Geometry: final body of the model. Coordinates: model frame, mm. A direction names the side the tool comes from. Round coordinates to 2 decimals unless told otherwise and drop trailing zeros. Write each loop counter-clockwise with the first axis right and the second up, starting at its lowest first coordinate (ties: lowest second). Pieces come first, ordered by that corner, then holes. Notation, with made-up numbers: M -5.5,8.25 L 19.5,8.25 A28 cw 19.5,32.25 Z; hole C -36.75,69 d9. An arc over 180 degrees is marked long. Answer as CSV lines item,"result". Start each with the question number.
Q1. Section query B-B on x = 9.75. Output: boundary loops of the cut face in (y, z), and give its area (3 significant figures).
Q2. First-contact query: pin 1 (1.6 mm diameter, centred on x = 5.5, y = 1.5, fed in from +Z); pin 2 (5 mm diameter, centred on x = 6.5, z = 3, fed in from +Y); pin 3 (6 mm diameter, centred on x = 6.5, z = 7.5, fed in from +Y); pin 4 (1.6 mm diameter, centred on y = 0.5, z = 6, fed in from +X). Flat tips, straight axial feed; report the tip coordinate or a pass-through.
Q3. Section query C-C on z = 12.5. Output: boundary loops of the cut face in (x, y).
Q4. Mould query, pull axis X, two halves, no side actions, for faces 1 (the flat face through (0, 0, 7)), 2 (the cylindrical face through (5.66, 0.89, 5.61)), 3 (the flat face through (7, 1.8, 7)). Classes: pulls with the +X half, pulls with the -X half, needs draft (parallel to the pull), parting line crosses it, or undercut.
Q5. Ray query, probe 1 along Z at (x, y) = (7, 0.3); probe 2 along Z at (x, y) = (10.5, 0.8); probe 3 along Y at (x, z) = (6, 1.75). Return the intervals inside material, ascending.
Q6. Reachability of faces 4 (the flat face through (1.5, 1, 7)), 5 (the flat face through (7, 1, 1.5)), 6 (the flat face through (6, 0, 6)) from +Z, -Z, +X, -X, +Y, -Y: full face, straight path, thin tool, end or side. Return the list, or none.
Q7. Section query D-D on y = -0.2. Output: boundary loops of the cut face in (x, z).
```python
from build123d import *

# Parameters (mm, degrees)
BOSS_EXTRUDE1_DEPTH = 1.2
BOSS_EXTRUDE2_DEPTH = 2
BOSS_EXTRUDE3_DEPTH = 1.8


with BuildPart() as part:
    # Sketch1 → Boss-Extrude1 (new body)
    with BuildSketch(Plane(origin=(0, 0, 0), x_dir=(1, 0, 0), z_dir=(0, 1, 0))):
        Polygon((0, 0), (14.45, 0), (0, -14.45), align=None)
    extrude(amount=-BOSS_EXTRUDE1_DEPTH)

    # Sketch2 → Boss-Extrude2 (add)
    with BuildSketch(Plane(origin=(0, 0, 0), x_dir=(1, 0, 0), z_dir=(0, 1, 0))):
        Polygon((0, 0), (14.45, 0), (12.95, -1.5), (1.5, -1.5), (1.5, -12.95), (0, -14.45), align=None)
    extrude(amount=BOSS_EXTRUDE2_DEPTH)

    # Sketch3 → Boss-Extrude3 (add)
    with BuildSketch(Plane(origin=(0, 0, 0), x_dir=(1, 0, 0), z_dir=(0, 1, 0))):
        with BuildLine():
            Line((4.997613639, -9.452386361), (9.452386361, -4.997613639))
            ThreePointArc((9.452386361, -4.997613639), (4.997613639, -4.997613639), (4.997613639, -9.452386361))
        make_face()
        with BuildLine():
            Line((5.13043724, -8.046770554), (8.046770554, -5.13043724))
            ThreePointArc((8.046770554, -5.13043724), (5.634009742, -5.634009742), (5.13043724, -8.046770554))
        make_face(mode=Mode.SUBTRACT)
    extrude(amount=BOSS_EXTRUDE3_DEPTH)


solid = part.part
```
Entries:
1,outline,"M -1.2,0 L 2,0 L 2,1.5 L 0,1.5 L 0,4.7 L -1.2,4.7 Z"
1,area,"8.64 mm^2"
2,pin 1,"stops at z = 9.45"
2,pin 2,"stops at y = 2"
2,pin 3,"stops at y = 1.8"
2,pin 4,"stops at x = 9.25"
3,outline,"M 0,-1.2 L 1.95,-1.2 L 1.95,0 L 1.5,0 L 1.5,2 L 0,2 Z"
4,face 1,"pulls with the -X half"
4,face 2,"undercut"
4,face 3,"needs draft"
5,probe 1,"z = 0 to 1.5, 4.08 to 4.99, 6.18 to 7.45"
5,probe 2,"z = 0 to 1.5"
5,probe 3,"y = -1.2 to 0"
6,face 4,"+Z, +Y"
6,face 5,"+X, +Y"
6,face 6,"+Y"
7,outline,"M 0,0 L 14.45,0 L 0,14.45 Z"
